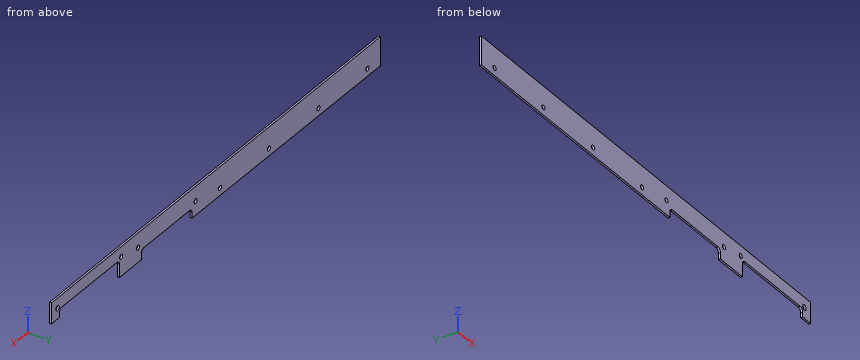
```python
from build123d import *

# Parameters (mm, degrees)
SKETCH_1_R      = 1.75
SKETCH_1_R_2    = 2
EXTRUDE_1_DEPTH = 1.5


with BuildPart() as part:
    # Эскиз1 → Бобышка-Вытянуть1 (new body)
    with BuildSketch(Plane(origin=(0, 0, 0), x_dir=(1, 0, 0), z_dir=(0, 1, 0))):
        with BuildLine():
            Line((299.3, 12.5), (299.3, 22.5))
            Line((299.3, 22.5), (274.05, 22.5))
            Line((274.05, 22.5), (274.05, 17.75))
            ThreePointArc((274.05, 17.75), (273.171320344, 15.628679656), (271.05, 14.75))
            Line((271.05, 14.75), (219.05, 14.75))
            ThreePointArc((219.05, 14.75), (216.928679656, 15.628679656), (216.05, 17.75))
            Line((216.05, 17.75), (216.05, 22))
            Line((216.05, 22), (0, 22))
            Line((0, 22), (0, 0))
            Line((0, 0), (377.3, 0))
            Line((377.3, 0), (377.3, 16))
            Line((377.3, 16), (368.3, 16))
            Line((368.3, 16), (368.3, 12.5))
            ThreePointArc((368.3, 12.5), (367.421320344, 10.378679656), (365.3, 9.5))
            Line((365.3, 9.5), (302.3, 9.5))
            ThreePointArc((302.3, 9.5), (300.178679656, 10.378679656), (299.3, 12.5))
        make_face()
        with Locations((212.05, 11.25)):
            Circle(SKETCH_1_R, mode=Mode.SUBTRACT)
        with Locations((278.05, 11.25)):
            Circle(SKETCH_1_R, mode=Mode.SUBTRACT)
        with Locations((297.3, 7.75)):
            Circle(SKETCH_1_R, mode=Mode.SUBTRACT)
        with Locations((370.3, 7.75)):
            Circle(SKETCH_1_R_2, mode=Mode.SUBTRACT)
        with Locations((15, 16.25)):
            Circle(SKETCH_1_R, mode=Mode.SUBTRACT)
        with Locations((71, 16.25)):
            Circle(SKETCH_1_R, mode=Mode.SUBTRACT)
        with Locations((128, 16.25)):
            Circle(SKETCH_1_R, mode=Mode.SUBTRACT)
        with Locations((184, 16.25)):
            Circle(SKETCH_1_R, mode=Mode.SUBTRACT)
    extrude(amount=EXTRUDE_1_DEPTH)


solid = part.part
```
Design review of the part built by this model. Coordinates are the model's own, in mm. Coordinates: 2 decimals unless noted, no trailing zeros. One line per item, written item: value. Start each with the question number.
Q1. For probe 1 along Z at (x, y) = (278.05, 0.6); probe 2 along X at (y, z) = (0.55, -11.25); probe 3 along X at (y, z) = (0.75, -16.25), list the stretches that pass through material, from the lowest coordinate up.
Q2. Insertion check: pin 1 Ø0.8 at (x, y) = (78.5, 0.5) entering from -Z; pin 2 Ø3 at (x, z) = (184, -16.25) entering from -Y; pin 3 Ø4 at (x, z) = (268.5, -15) entering from -Y. Each pin has a flat end and moves straight along its axis. Give the tip position at first contact, or say it passes through.
Q3. Take a section at A-A, the plane y = 0.7. Give the number of separate pieces and of enclosed holes in the cut face, then the cut area to 3 significant figures.
Values follow:
1. probe 1: z = -22.5 to -13, -9.5 to 0
1. probe 2: x = 0 to 210.3, 213.8 to 276.3, 279.8 to 299.57, 368.03 to 377.3
1. probe 3: x = 0 to 13.25, 16.75 to 69.25, 72.75 to 126.25, 129.75 to 182.25, 185.75 to 216.45, 273.65 to 299.3
2. pin 1: stops at z = -22
2. pin 2: passes through
2. pin 3: stops at y = 0
3. separate pieces: 1
3. enclosed holes: 8
3. area: 6,900 mm2
